```python
from build123d import *

# Parameters (mm, degrees)
BOSS_EXTRUDE1_START   = 5
SKETCH1_R             = 30
BOSS_EXTRUDE1_DEPTH   = 32.5
BOSS_EXTRUDE1_2_DEPTH = 32.5
SKETCH1_3_ONE_SIDE_W  = 196.833752096
SKETCH1_3_ONE_SIDE_H  = 25
CUT_EXTRUDE1_START    = 37.5
SKETCH1_4_R           = 15
CUT_EXTRUDE1_DEPTH    = 15
BOSS_EXTRUDE2_START   = 37.5
SKETCH1_5_R           = 15
BOSS_EXTRUDE2_DEPTH   = 15


with BuildPart() as part:
    # Sketch1 → Boss-Extrude1 (new body, symmetric)
    with BuildSketch(Plane.XY.offset(BOSS_EXTRUDE1_START)):
        Circle(SKETCH1_R)
    extrude(amount=BOSS_EXTRUDE1_DEPTH, both=True)



with BuildPart() as body_2:
    # Sketch1 → Boss-Extrude1 2 (new body, symmetric)
    with BuildSketch(Plane.XY.offset(BOSS_EXTRUDE1_START)):
        with Locations((230, 0)):
            Circle(SKETCH1_R)
    extrude(amount=BOSS_EXTRUDE1_2_DEPTH, both=True)


with BuildPart() as part_1:
    add(part.part)

    add(body_2.part)  # Revolve1 merges body 2
    # Sketch1<3> one side → Revolve1 (revolve)
    with BuildSketch(Plane.XY):
        with Locations((115, 12.5)):
            Rectangle(SKETCH1_3_ONE_SIDE_W, SKETCH1_3_ONE_SIDE_H)
    revolve(axis=Axis((213.416876048, 0, 0), (-1, 0, 0)))

    # Sketch1<4> → Cut-Extrude1 (cut)
    with BuildSketch(Plane.XY.offset(CUT_EXTRUDE1_START)):
        Circle(SKETCH1_4_R)
    extrude(amount=-CUT_EXTRUDE1_DEPTH, mode=Mode.SUBTRACT)

    # Sketch1<5> → Boss-Extrude2 (add)
    with BuildSketch(Plane.XY.offset(BOSS_EXTRUDE2_START)):
        with Locations((230, 0)):
            Circle(SKETCH1_5_R)
    extrude(amount=BOSS_EXTRUDE2_DEPTH)


solid = part_1.part
```
The model under review builds one solid part; all positions refer to its coordinate system, in mm. A direction names the side the tool comes from. Round coordinates to 2 decimals unless told otherwise and drop trailing zeros. Order: outer loops, then holes, each group sorted by start corner. A loop starts at its lowest first (then second) coordinate and runs counter-clockwise, first axis right, second up. Notation, with made-up numbers: (31, 42.5) -> (79, 42.5) arc R10 cw to (79, 55.5) -> close; hole circle Ø7 at (67.5, -26.75). An arc over 180 degrees is marked (long way). One line per item, written item: value. Start each with the question number.
Q1. Mouldability with a two-part tool opening along X and no side actions: class faces 1 (the face through (244.307, 4.506, 44.895)), 2 (the face through (116.378, -24.976, -1.099)), 3 (the face through (230, 0, -27.5)) as released by +X, released by -X, zero draft, split by the parting line, or undercut.
Q2. Clearance check with flat-ended pins moving along their axes: pin 1 Ø24 at (x, y) = (-2, -6.5) entering from +Z; pin 2 Ø1 at (y, z) = (-1, 24.5) entering from +X; pin 3 Ø6 at (x, z) = (138.5, -9) entering from +Y. State where each tip first meets the part, or that it passes through.
Q3. Wall thickness on line 1 (Y direction, x = 0, z = 32.5); line 2 (Z direction, x = 15, y = 25.5); line 3 (Z direction, x = 205.5, y = -20): over which ranges is each line inside the solid? List them lowest first.
Q4. Machinability: for faces 4 (the face through (216, -6, 37.5)), 5 (the face through (0, 0, -27.5)), 6 (the face through (6, 14, 37.5)), which of the approach directions +Z, -Z, +X, -X, +Y, -Y give a long, thin tool a straight path to every point of the face, cutting with its end or side? Answer none if there is none.
Q5. Take a section at B-B (z = 33.5). Write out the cut boundary in (x, y).
Q6. Take a section at A-A (y = 0). Write out the cut boundary in (x, z), and give its area (3 significant figures).
Q7. Take a section at D-D (z = 0). Write out the cut boundary in (x, y), and give its area (3 significant figures).
Q8. Take a section at C-C (x = 230). Write out the cut boundary in (y, z).
Reported:
1. face 1: split by the parting line
1. face 2: undercut
1. face 3: zero draft
2. pin 1: stops at z = 37.5
2. pin 2: stops at x = 260
2. pin 3: stops at y = 24.27
3. line 1: y = -30 to -15, 15 to 30
3. line 2: z = -27.5 to 37.5
3. line 3: z = -15 to 15
4. face 4: +Z
4. face 5: -Z, +X, -X, +Y, -Y
4. face 6: +Z, -X, +Y, -Y
5. outline: circle Ø60 at (0, 0); circle Ø60 at (230, 0); hole circle Ø30 at (0, 0)
6. outline: (-30, -27.5) -> (30, -27.5) -> (30, -25) -> (200, -25) -> (200, -27.5) -> (260, -27.5) -> (260, 37.5) -> (245, 37.5) -> (245, 52.5) -> (215, 52.5) -> (215, 37.5) -> (200, 37.5) -> (200, 25) -> (30, 25) -> (30, 37.5) -> (15, 37.5) -> (15, 22.5) -> (-15, 22.5) -> (-15, 37.5) -> (-30, 37.5) -> close
6. area: 16,300 mm2
7. outline: (16.58, -25) -> (213.42, -25) arc R30 ccw (long way) to (213.42, 25) -> (16.58, 25) arc R30 ccw (long way) to start
7. area: 14,600 mm2
8. outline: (-30, -27.5) -> (30, -27.5) -> (30, 37.5) -> (15, 37.5) -> (15, 52.5) -> (-15, 52.5) -> (-15, 37.5) -> (-30, 37.5) -> close
